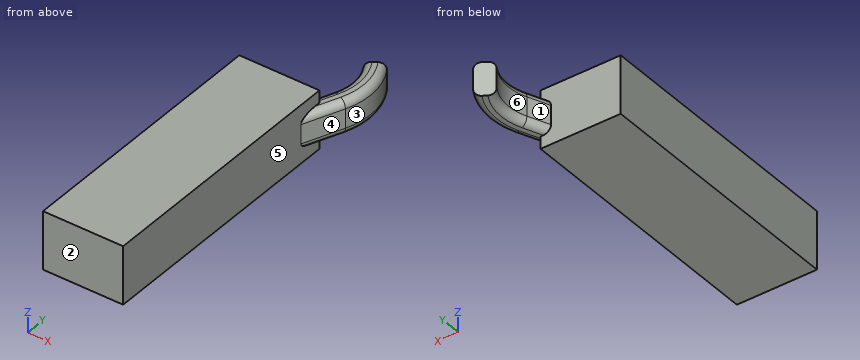
from build123d import *

# Parameters (mm, degrees)
SKETCH1_W   = 33.5
SKETCH1_H   = 110.5
BODY_DEPTH  = 12.15
CABLE_DEPTH = 7
FILLET1_R   = 3


with BuildPart() as part:
    # Sketch1 → Body (new, symmetric)
    with BuildSketch(Plane.XY):
        Rectangle(SKETCH1_W, SKETCH1_H)
    extrude(amount=BODY_DEPTH, both=True)

    # Sketch2 → Cable (add, symmetric)
    with BuildSketch(Plane.XY):
        with BuildLine():
            Line((14.614768377, 39.692127969), (23.378177187, 60.932254406))
            ThreePointArc((23.378177187, 60.932254406), (25.480222235, 74.274540457), (21.310589844, 87.121694079))
            Line((21.310589844, 87.121694079), (14.485707158, 82.94784977))
            ThreePointArc((14.485707158, 82.94784977), (17.505037046, 73.644920573), (15.98289628, 63.98345422))
            Line((15.98289628, 63.98345422), (7.21948747, 42.743327783))
            Line((7.21948747, 42.743327783), (14.614768377, 39.692127969))
        make_face()
    extrude(amount=CABLE_DEPTH, both=True)

    # Fillet1
    fillet1_edges = [part.edges().sort_by_distance(p)[0] for p in [
        (20.064088593, 52.899802391, -7),
        (14.18123964, 59.61672711, 7),
        (20.064088593, 52.899802391, 7),
        (25.480222235, 74.274540457, 7),
        (14.18123964, 59.61672711, -7),
        (17.505037046, 73.644920573, -7),
        (25.480222235, 74.274540457, -7),
        (17.505037046, 73.644920573, 7),
    ]]
    fillet(fillet1_edges, radius=FILLET1_R)


solid = part.part
Part model, mm, in its own coordinate system. Face numbers are marked on the shaded views. A direction names the side the tool comes from. Give positions to 0.01 mm unless a question says otherwise; leave off trailing zeros. Loops run counter-clockwise (first coordinate to the right, second up) from the corner with the lowest first, then second, coordinate; pieces in that order, holes last. Notation, with made-up numbers: M -3,-36 L 7,-36 A21 cw 7,-24 Z; hole C 13.25,-36 d8. An arc over 180 degrees is marked long. Put each result on its own line as item: value. Start each with the question number.
1) Probe probe 1 along X at (y, z) = (35, -10); probe 2 along Y at (x, z) = (3, 8); probe 3 along Z at (x, y) = (21, 80). List the from-to ranges inside material, lowest first.
2) Flat gauge pins, fed straight in: pin 1 (8 mm diameter, centred on x = -11, z = -4, fed in from +Y); pin 2 (2 mm diameter, centred on x = 18, y = 70.5, fed in from -Z); pin 3 (7.5 mm diameter, centred on y = -17, z = -1, fed in from +X). Where does each tip first touch, or does it go through?
3) Pull direction Y, two halves, no side cores. Call the marked faces 3, 4, 5 and 6: +Y half, -Y half, draft (parallel to the pull), parting line (faces both ways), or undercut.
4) Saw through at D-D (z = 5.5). List the corners of the cut face in (x, y), then the cut area to 3 significant figures.
5) Saw through at C-C (y = 11.5). List the corners of the cut face in (x, z).
6) Saw through at A-A (z = -1). List the corners of the cut face in (x, y).
7) Saw through at B-B (x = 3.5). List the corners of the cut face in (y, z).
8) 3-axis set-ups, long thin cutter, end or side, ignore diameter. For the marked faces 1 and 2: which of +Z, -Z, +X, -X, +Y, -Y reach the whole face in a straight line?
Numbers:
1. probe 1: -16.75 to 16.75
1. probe 2: -55.25 to 55.25
1. probe 3: -7 to 7
2. pin 1: y = 55.25
2. pin 2: z = -6.59
2. pin 3: x = 16.75
3. face 3: parting line
3. face 4: -Y half
3. face 5: draft
3. face 6: undercut
4. outline: M -16.75,-55.25 L 16.75,-55.25 L 16.75,45.92 L 23.01,61.09 A28.6 ccw 20.97,86.91 L 14.83,83.16 A21.4 cw 16.35,63.83 L 12.81,55.25 L -16.75,55.25 Z
4. area: 3,940 mm^2
5. outline: M -16.75,-12.15 L 16.75,-12.15 L 16.75,12.15 L -16.75,12.15 Z
6. outline: M -16.75,-55.25 L 16.75,-55.25 L 16.75,44.87 L 23.38,60.93 A29 ccw 21.31,87.12 L 14.49,82.95 A21 cw 15.98,63.98 L 12.38,55.25 L -16.75,55.25 Z
7. outline: M -55.25,-12.15 L 55.25,-12.15 L 55.25,12.15 L -55.25,12.15 Z
8. face 1: +Z, -Z, -X
8. face 2: +Z, -Z, +X, -X, -Y
